Print and shaded views of the part. All mm, measured from the part's lowest x, y and z. Give positions to 0.01 mm unless a question says otherwise; leave off trailing zeros. Order: outer loops, then holes, each group sorted by start corner. A loop starts at its lowest first (then second) coordinate and runs counter-clockwise, first axis right, second up. Notation, with made-up numbers: (-29.5, 20) - (2.5, 20) arc R18 cw to (2.5, 49) - close; hole circle Ø3 at (-9, 42.5). An arc over 180 degrees is marked (long way). Answer in a Markdown table with one row per item.
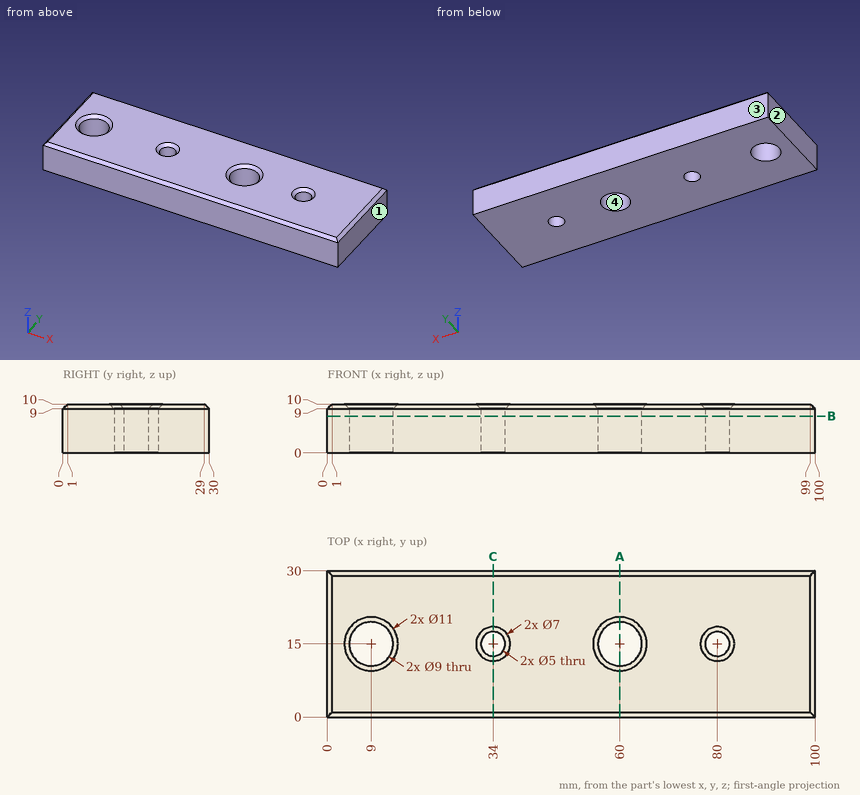
1. Two-plate mould, pull along X, no slides. Class the marked faces 1, 2, 3 and 4: +X half, -X half, draft (parallel to the pull), parting line (faces both ways), or undercut.
Check result:
| item | result |
|---|---|
| face 1 | +X half |
| face 2 | -X half |
| face 3 | draft |
| face 4 | undercut |
2. Cut at B-B on z = 7.5. Write the cut outline in (x, y).
Check result:
| item | result |
|---|---|
| outline | (0, 0) - (100, 0) - (100, 30) - (0, 30) - close; hole circle Ø9 at (9, 15); hole circle Ø5 at (34, 15); hole circle Ø9 at (60, 15); hole circle Ø5 at (80, 15) |
3. Probe line 1 (Y direction, x = 34, z = 4.5); line 2 (X direction, y = 18, z = 5); line 3 (X direction, y = 11.5, z = 7.5). List the from-to ranges inside material, lowest first.
Check result:
| item | result |
|---|---|
| line 1 | y = 0 to 12.5, 17.5 to 30 |
| line 2 | x = 0 to 5.65, 12.35 to 56.65, 63.35 to 100 |
| line 3 | x = 0 to 6.17, 11.83 to 57.17, 62.83 to 100 |
4. Cut at A-A on x = 60. Write the cut outline in (y, z).
Check result:
| item | result |
|---|---|
| outline | (0, 0) - (10.5, 0) - (10.5, 9) - (9.5, 10) - (1, 10) - (0, 9) - close; (19.5, 0) - (30, 0) - (30, 9) - (29, 10) - (20.5, 10) - (19.5, 9) - close |
5. Cut at C-C on x = 34. Write the cut outline in (y, z).
Check result:
| item | result |
|---|---|
| outline | (0, 0) - (12.5, 0) - (12.5, 9) - (11.5, 10) - (1, 10) - (0, 9) - close; (17.5, 0) - (30, 0) - (30, 9) - (29, 10) - (18.5, 10) - (17.5, 9) - close |
6. Drop flat-ended pins along their axis: P1, Ø7, axis at x = 9, y = 15, coming from the -Z side; P2, Ø8, axis at x = 36, y = 4.5, coming from the -Z side. Give the stop position or say it passes through.
Check result:
| item | result |
|---|---|
| P1 | passes through |
| P2 | stops at z = 0 |
